from build123d import *

# Parameters (mm, degrees)
SKETCH_1_R          = 7.35
EXTRUDE_1_DEPTH     = 3.3
SKETCH_2_R          = 3
EXTRUDE_342_DEPTH   = 28
SKETCH_3_R          = 14.8
EXTRUDE_3_DEPTH     = 9.2
FILLET_1_R          = 4
SKETCH_4_R          = 5
CUT_EXTRUDE_1_DEPTH = 10


with BuildPart() as part:
    # Эскиз1 → Бобышка-Вытянуть1 (new body)
    with BuildSketch(Plane(origin=(0, 0, 0), x_dir=(1, 0, 0), z_dir=(0, 1, 0))):
        with Locations(Location((0, 0, 0), (0, 0, 270))):
            Circle(SKETCH_1_R)
    extrude(amount=EXTRUDE_1_DEPTH)

    # Эскиз2 → Extrude 342 (add)
    with BuildSketch(Plane.XZ):
        with Locations(Location((0, 0, 0), (0, 0, 270))):
            Circle(SKETCH_2_R)
    extrude(amount=EXTRUDE_342_DEPTH)

    # Эскиз3 → Бобышка-Вытянуть3 (add)
    with BuildSketch(Plane(origin=(0, 3.3, 0), x_dir=(1, 0, 0), z_dir=(0, 1, 0))):
        with Locations(Location((0, 0, 0), (0, 0, 270))):
            Circle(SKETCH_3_R)
    extrude(amount=EXTRUDE_3_DEPTH)

    # Скругление1
    fillet_1_edges = [part.edges().sort_by_distance(p)[0] for p in [
        (0, 12.5, -14.8),
    ]]
    fillet(fillet_1_edges, radius=FILLET_1_R)

    # Эскиз4 → Вырез-Вытянуть1 (cut)
    with BuildSketch(Plane(origin=(0, 12.5, 0), x_dir=(1, 0, 0), z_dir=(0, 1, 0))):
        with Locations((0, 18)):
            Circle(SKETCH_4_R)
        with Locations((15.588457268, 9)):
            Circle(SKETCH_4_R)
        with Locations((15.588457268, -9)):
            Circle(SKETCH_4_R)
        with Locations((0, -18)):
            Circle(SKETCH_4_R)
        with Locations((-15.588457268, -9)):
            Circle(SKETCH_4_R)
        with Locations((-15.588457268, 9)):
            Circle(SKETCH_4_R)
    extrude(amount=-CUT_EXTRUDE_1_DEPTH, mode=Mode.SUBTRACT)


solid = part.part
Check sheet for the modelled part. Datum: model origin and axes. Units: mm. A direction names the side the tool comes from. Round coordinates to 2 decimals unless told otherwise and drop trailing zeros. Loops run counter-clockwise (first coordinate to the right, second up) from the corner with the lowest first, then second, coordinate; pieces in that order, holes last.
1. Sectioned sample at A-A on x = 0. Record the boundary of the cut face in (y, z).
2. Sectioned sample at C-C on y = 6.5. Record the boundary of the cut face in (x, z), and give its area (3 significant figures).
3. Sectioned sample at D-D on y = -20.5. Record the boundary of the cut face in (x, z), and give its area (3 significant figures).
4. Set-up check for faces 1 (the flat face through (-3.2, 0, -0.1)), 2 (the cylindrical face through (-7.348, 5.864, -12.847)): record each of +Z, -Z, +X, -X, +Y, -Y from which the full face is reachable in a straight line by a thin tool's end or side.
5. Mould release check, pull along Z, two halves, no side actions. Record for faces 3 (the cylindrical face through (-11.23, 7.63, 6.55)), 4 (the flat face through (0, -28, 0)), 5 (the cylindrical face through (-7.175, 1.627, -1.593)): released by +Z, released by -Z, zero draft, split by the parting line, or undercut.
6. Sectioned sample at B-B on z = 0. Record the boundary of the cut face in (x, y).
7. Gauge pin test, flat ends, axial feed: pin 1 Ø8 at (x, y) = (-0.5, -13.5) entering from -Z; pin 2 Ø1.5 at (y, z) = (5.5, -4.5) entering from +X; pin 3 Ø4 at (x, y) = (3.5, -6) entering from +Z; pin 4 Ø10 at (x, y) = (10, -12.5) entering from -Z. Record the tip position at first contact, or that the pin passes through.
8. Scan lines: probe 1 along Y at (x, z) = (5.25, -4.75); probe 2 along Y at (x, z) = (-8.25, 2); probe 3 along Z at (x, y) = (-7.5, 10.5). Record each from-to range of solid material in increasing order.
Recorded:
1. outline: (-28, -3) - (0, -3) - (0, -7.35) - (3.3, -7.35) - (3.3, -13) - (11.84, -13) arc R4 ccw to (12.5, -10.8) - (12.5, 10.8) arc R4 ccw to (11.84, 13) - (3.3, 13) - (3.3, 7.35) - (0, 7.35) - (0, 3) - (-28, 3) - close
2. outline: (-14.19, -4.2) arc R5 cw to (-10.73, -10.19) arc R14.8 ccw to (-3.46, -14.39) arc R5 cw to (3.46, -14.39) arc R14.8 ccw to (10.73, -10.19) arc R5 cw to (14.19, -4.2) arc R14.8 ccw to (14.19, 4.2) arc R5 cw to (10.73, 10.19) arc R14.8 ccw to (3.46, 14.39) arc R5 cw to (-3.46, 14.39) arc R14.8 ccw to (-10.73, 10.19) arc R5 cw to (-14.19, 4.2) arc R14.8 ccw to start
2. area: 637 mm2
3. outline: circle Ø6 at (0, 0)
3. area: 28.3 mm2
4. face 1: -Y
4. face 2: -Z, -X, +Y, -Y
5. face 3: undercut
5. face 4: zero draft
5. face 5: split by the parting line
6. outline: (-14.8, 3.3) - (-7.35, 3.3) - (-7.35, 0) - (-3, 0) - (-3, -28) - (3, -28) - (3, 0) - (7.35, 0) - (7.35, 3.3) - (14.8, 3.3) - (14.8, 8.5) arc R4 ccw to (10.8, 12.5) - (-10.8, 12.5) arc R4 ccw to (-14.8, 8.5) - close
7. pin 1: stops at z = -3
7. pin 2: stops at x = 14.32
7. pin 3: stops at z = 2.6
7. pin 4: passes through
8. probe 1: y = 0 to 12.5
8. probe 2: y = 3.3 to 12.5
8. probe 3: z = -12.13 to 12.13
